```python
from build123d import *
from build123d.topology import SkipClean

# Parameters (mm, degrees)
CUT_SWEEP1_PITCH = 1.27


with BuildPart() as part:
    # Sketch1 → Revolve1 (revolve)
    with BuildSketch(Plane.XY, mode=Mode.PRIVATE) as revolve1_sk:
        Polygon((-13.0937, 8.6614), (-13.0937, 7.4803), (-6.065803329, 2.1844), (13.0937, 2.1844), (13.0937, 2.51206), (13.0937, 5.55625), (9.053923424, 5.55625), (-0.8763, 5.55625), (-0.8763, 7.1374), (-7.5311, 7.1374), (-7.5311, 8.6614), align=None)
    revolve(revolve1_sk.sketch.rotate(Axis((-13.0937, 0, 0), (1, 0, 0)), 90), axis=Axis((-13.0937, 0, 0), (1, 0, 0)))

    # Cut-Sweep1: the profile of Sketch4 profile screwed along a right-hand helix of 11 turns, 8 arcs to a turn; built about Z, then put on its axis
    cut_sweep1_z = Axis((0, 0, 0), (0, 0, 1))
    cut_sweep1_corners = [(5.55655, 0, 0.000173205), (5.55655, 0, -1.111423205), (4.731360803, 0, -0.635), (4.731360803, 0, -0.47625)]
    with BuildLine(mode=Mode.PRIVATE) as cut_sweep1_profile:
        Line(cut_sweep1_corners[0], cut_sweep1_corners[1])
        Line(cut_sweep1_corners[1], cut_sweep1_corners[2])
        Line(cut_sweep1_corners[2], cut_sweep1_corners[3])
        Line(cut_sweep1_corners[3], cut_sweep1_corners[0])
    cut_sweep1_cap = Face(cut_sweep1_profile.wire())
    cut_sweep1_turn_angles = [0, 22.5, 45, 67.5, 90, 112.5, 135, 157.5, 180, 202.5, 225, 247.5, 270, 292.5, 315, 337.5, 360]
    cut_sweep1_turn_weights = [1, 0.9238795325112867, 1, 0.9238795325112867, 1, 0.9238795325112867, 1, 0.9238795325112867, 1, 0.9238795325112867, 1, 0.9238795325112867, 1, 0.9238795325112867, 1, 0.9238795325112867, 1]
    cut_sweep1_turn_rails = [Edge.make_bspline([Vector(p[0], p[1], 0).rotate(cut_sweep1_z, cut_sweep1_turn_angles[k]) / cut_sweep1_turn_weights[k] + Vector(0, 0, p[2] + CUT_SWEEP1_PITCH * cut_sweep1_turn_angles[k] / 360) for k in range(17)], [0, 0, 0, 1, 1, 2, 2, 3, 3, 4, 4, 5, 5, 6, 6, 7, 7, 8, 8, 8], 2, cut_sweep1_turn_weights) for p in cut_sweep1_corners]
    cut_sweep1_turn_sides = [Face.make_surface_from_curves(cut_sweep1_turn_rails[p[0]], cut_sweep1_turn_rails[p[1]]) for p in [(0, 1), (1, 2), (2, 3), (3, 0)]]
    cut_sweep1_turn = Solid(Shell([*cut_sweep1_turn_sides, cut_sweep1_cap, cut_sweep1_cap.rotate(cut_sweep1_z, 360).moved(Location((0, 0, CUT_SWEEP1_PITCH * 360 / 360)))]))
    cut_sweep1_each = [*[cut_sweep1_turn.moved(Location((0, 0, CUT_SWEEP1_PITCH * i))) for i in range(11)]]
    add(Plane(origin=(13.0937, 0, 0), x_dir=(0, 1, 0), z_dir=(-1, 0, 0)) * Compound([cut_sweep1_each[i] for i in range(0, 11, 2)]), mode=Mode.SUBTRACT)
    add(Plane(origin=(13.0937, 0, 0), x_dir=(0, 1, 0), z_dir=(-1, 0, 0)) * Compound([cut_sweep1_each[i] for i in range(1, 11, 2)]), mode=Mode.SUBTRACT)

    # Sketch5 → Cut-Revolve1 (revolve, cut)
    with BuildSketch(Plane.XY, mode=Mode.PRIVATE) as cut_revolve1_sk:
        Polygon((13.0937, 2.51206), (10.216002239, 4.680560803), (8.946002239, 4.680560803), (8.070313042, 5.55625), (13.0937, 5.55625), align=None)
        Polygon((-0.8763, 5.55625), (-0.8763, 4.680560803), (0.3937, 4.680560803), (1.269389197, 5.55625), align=None)
    revolve(cut_revolve1_sk.sketch.rotate(Axis((0, 0, 0), (-1, 0, 0)), 90), axis=Axis((0, 0, 0), (-1, 0, 0)), mode=Mode.SUBTRACT)

    # Sketch6 → Revolve2 (revolve)
    with SkipClean():  # the faces are left unmerged after this step: merging them gives an invalid solid
        with BuildSketch(Plane.XY, mode=Mode.PRIVATE) as revolve2_sk:
            Polygon((1.269389197, 5.55625), (0.3937, 4.680560803), (8.946002239, 4.680560803), (8.070313042, 5.55625), align=None)
        revolve(revolve2_sk.sketch.rotate(Axis((0, 0, 0), (-1, 0, 0)), 90), axis=Axis((0, 0, 0), (-1, 0, 0)))
    add(part.part.scale(1), mode=Mode.REPLACE)  # the faces are merged on a copy


solid = part.part
```
The model under review builds one solid part; all positions refer to its coordinate system, in mm. A direction names the side the tool comes from. Round coordinates to 2 decimals unless told otherwise and drop trailing zeros. Loops run counter-clockwise (first coordinate to the right, second up) from the corner with the lowest first, then second, coordinate; pieces in that order, holes last. Notation, with made-up numbers: M 32,0.5 L 78,0.5 A8 cw 78,9.5 Z; hole C -33.75,14 d10. An arc over 180 degrees is marked long. Answer as a JSON object with one key per item and string values.
(1) Take a section at B-B on x = -11. Give the boundary of the cut face in (y, z), and give its area (3 significant figures).
Resolved:
{"outline": "C 0,0 d17.32; hole C 0,0 d11.81", "area": "126 mm²"}
(2) Tool access review of faces 1 (the cylindrical face through (-10.351, 7.684, 3.997)), 2 (the flat face through (-0.876, 5, -1)), 3 (the cylindrical face through (-4.25, -0.31, -7.13)): name each direction out of +Z, -Z, +X, -X, +Y, -Y from which nothing blocks a thin tool from reaching the whole face with its end or side.
Resolved:
{"face 1": "+X, -X", "face 2": "none", "face 3": "+X"}
(3) Draft analysis for pull direction Y (two halves, no side actions). For faces 4 (the cylindrical face through (3.648, -0.656, 2.084)), 5 (the flat face through (-7.531, -7.1, -1.9)), 6 (the cylindrical face through (-0.232, -1.406, -4.464)), state which applies: released by +Y, released by -Y, zero draft, split by the parting line, or undercut.
Resolved:
{"face 4": "undercut", "face 5": "zero draft", "face 6": "split by the parting line"}
(4) Take a section at A-A on x = -5.75. Give the boundary of the cut face in (y, z), and give its area (3 significant figures).
Resolved:
{"outline": "C 0,0 d14.27; hole C 0,0 d4.37", "area": "145 mm²"}
(5) To check wall thickness, follow line 1 along Y through (x, z) = (4, 0); line 2 along X through (y, z) = (5.5, 5.5); line 3 along Z through (x, y) = (-2.5, -2). State the ranges of each line that lie inside material, in increasing order.
Resolved:
{"line 1": "-5.56 to -2.18, 2.18 to 5.56", "line 2": "-13.09 to -7.53", "line 3": "-6.85 to -0.88, 0.88 to 6.85"}
(6) Clearance check with flat-ended pins moving along their axes: P1, Ø4, axis at y = 0, z = 0, coming from the +X side; P2, Ø1.5, axis at y = -1, z = -5.5, coming from the -X side; P3, Ø1, axis at x = 10, z = -2, coming from the +Y side; P4, Ø3, axis at x = 9, y = 3, coming from the -Z side. State where each tip first meets the part, or that it passes through.
Resolved:
{"P1": "through", "P2": "x = -11.58", "P3": "y = 4.43", "P4": "z = -5.25"}
